Work out the finished part from the listing and answer in its coordinate system (mm). Round coordinates to 2 decimals unless told otherwise and drop trailing zeros. Write each loop counter-clockwise with the first axis right and the second up, starting at its lowest first coordinate (ties: lowest second). Pieces come first, ordered by that corner, then holes.
1. Find section A-A (z = -5). Write down the section's boundary in (x, y).
2. Find section C-C (x = 12). Write down the section's boundary in (y, z).
3. Flat-ended cylindrical pins translate along their axes: pin 1 Ø2.5 at (x, z) = (-12.5, -99.5) entering from -Y; pin 2 Ø3.5 at (x, z) = (12.5, -99.5) entering from +Y. Find the tip coordinate at first contact, or state that the pin passes through.
4. Straight lines are drawn through the part: probe 1 along X at (y, z) = (0.8, -5); probe 2 along X at (y, z) = (1.85, -99.5); probe 3 along Z at (x, y) = (1, 2.55). For each, find the intervals that lie inside material, in ascending order.
5. Find section B-B (y = 0.8). Write down the section's boundary in (x, z).
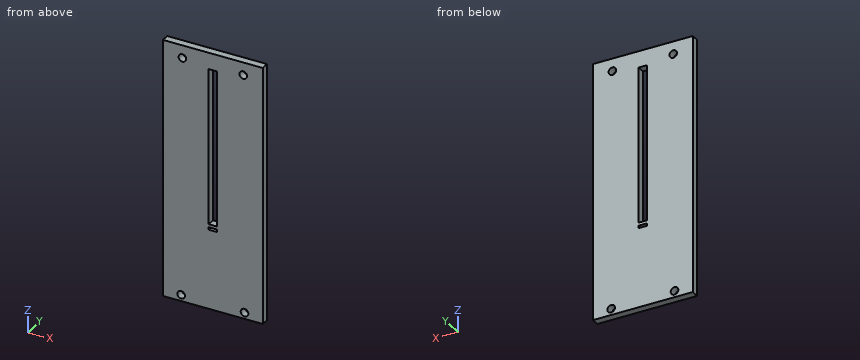
```python
from build123d import *

# Parameters (mm, degrees)
SKETCH1_W             = 39.4
SKETCH1_H             = 102
BOSS_EXTRUDE1_DEPTH   = 3.05
SKETCH4_W             = 1.65
SKETCH4_H             = 1
SKETCH4_H_2           = 61.8
CUT_EXTRUDE1_DEPTH    = 104.929747907
SKETCH7_R             = 1.5
CUT_EXTRUDE4_DEPTH    = 104.929747907
F_3_0MM_DOWEL_HOLE1_D = 3


with BuildPart() as part:
    # Sketch1 → Boss-Extrude1 (new body)
    with BuildSketch(Plane(origin=(0, 0, 0), x_dir=(1, 0, 0), z_dir=(0, 1, 0))):
        with Locations((0, 51)):
            Rectangle(SKETCH1_W, SKETCH1_H)
    extrude(amount=BOSS_EXTRUDE1_DEPTH)

    # Sketch4 → Cut-Extrude1 (cut, through all)
    with BuildSketch(Plane(origin=(0, 3.05, 0), x_dir=(1, 0, 0), z_dir=(0, 1, 0))):
        with Locations((-0.825, 70)):
            Rectangle(SKETCH4_W, SKETCH4_H)
        with Locations((-0.825, 37.4)):
            Rectangle(SKETCH4_W, SKETCH4_H_2)
        with Locations((0.825, 37.4)):
            Rectangle(SKETCH4_W, SKETCH4_H_2)
        with Locations((0.825, 70)):
            Rectangle(SKETCH4_W, SKETCH4_H)
    extrude(amount=-CUT_EXTRUDE1_DEPTH, mode=Mode.SUBTRACT)

    # Sketch7 → Cut-Extrude4 (cut, through all)
    with BuildSketch(Plane(origin=(0, 3.05, 0), x_dir=(1, 0, 0), z_dir=(0, 1, 0))):
        with Locations(Location((-12, 5, 0), (0, 0, 270))):
            Circle(SKETCH7_R)
        with Locations(Location((12, 5, 0), (0, 0, 90))):
            Circle(SKETCH7_R)
    extrude(amount=-CUT_EXTRUDE4_DEPTH, mode=Mode.SUBTRACT)

    # Ø3.0mm Dowel Hole1 (through all)
    with Locations(Plane(origin=(0, 3.05, 0), x_dir=(1, 0, 0), z_dir=(0, 1, 0))):
        with Locations((-12.5, 99.5), (12.5, 99.5)):
            Hole(F_3_0MM_DOWEL_HOLE1_D / 2)


solid = part.part
```
Worked answers:
1. outline: (-19.7, 0) - (-13.5, 0) - (-13.5, 3.05) - (-19.7, 3.05) - close; (-10.5, 0) - (10.5, 0) - (10.5, 3.05) - (-10.5, 3.05) - close; (13.5, 0) - (19.7, 0) - (19.7, 3.05) - (13.5, 3.05) - close
2. outline: (0, -102) - (3.05, -102) - (3.05, -100.91) - (0, -100.91) - close; (0, -98.09) - (3.05, -98.09) - (3.05, -6.5) - (0, -6.5) - close; (0, -3.5) - (3.05, -3.5) - (3.05, 0) - (0, 0) - close
3. pin 1: passes through
3. pin 2: stops at y = 3.05
4. probe 1: x = -19.7 to -13.5, -10.5 to 10.5, 13.5 to 19.7
4. probe 2: x = -19.7 to -14, -11 to 11, 14 to 19.7
4. probe 3: z = -102 to -70.5, -69.5 to -68.3, -6.5 to 0
5. outline: (-19.7, -102) - (19.7, -102) - (19.7, 0) - (-19.7, 0) - close; hole circle Ø3 at (-12.5, -99.5); hole circle Ø3 at (-12, -5); hole (-1.65, -70.5) - (1.65, -70.5) - (1.65, -69.5) - (-1.65, -69.5) - close; hole (-1.65, -68.3) - (1.65, -68.3) - (1.65, -6.5) - (-1.65, -6.5) - close; hole circle Ø3 at (12, -5); hole circle Ø3 at (12.5, -99.5)
